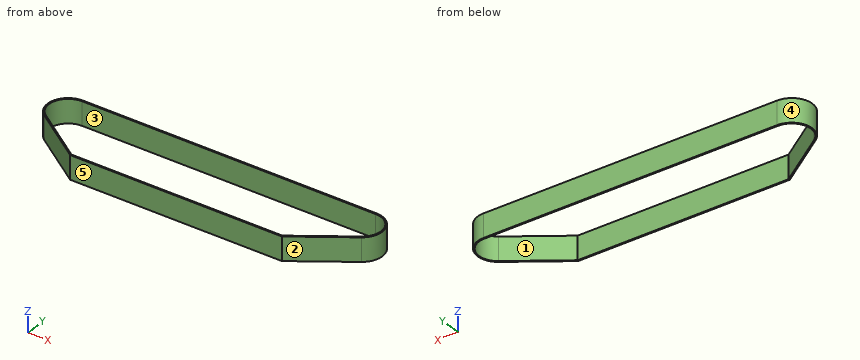
```python
from build123d import *

# Parameters (mm, degrees)
EXTRUDE_1_DEPTH = 35


with BuildPart() as part:
    # 草图1 → 拉伸-薄壁1 (new body)
    with BuildSketch(Plane.XY):
        with BuildLine():
            Line((237.450135309, -25.014851143), (158.628665481, -80))
            Line((158.628665481, -80), (-158.628665481, -80))
            Line((-158.628665481, -80), (-237.450135309, -25.014851143))
            ThreePointArc((-237.450135309, -25.014851143), (-249.09641696, 9.145956487), (-220, 30.5))
            Line((-220, 30.5), (220, 30.5))
            ThreePointArc((220, 30.5), (249.09641696, 9.145956487), (237.450135309, -25.014851143))
        make_face()
        with BuildLine():
            Line((236.305864141, -23.374533035), (158, -78))
            Line((158, -78), (-158, -78))
            Line((-158, -78), (-236.305864141, -23.374533035))
            ThreePointArc((-236.305864141, -23.374533035), (-247.188455192, 8.546221636), (-220, 28.5))
            Line((-220, 28.5), (220, 28.5))
            ThreePointArc((220, 28.5), (247.188455192, 8.546221636), (236.305864141, -23.374533035))
        make_face(mode=Mode.SUBTRACT)
    extrude(amount=EXTRUDE_1_DEPTH)


solid = part.part
```
Input: part model. Units: mm. Frame: model coordinates. Face numbers are marked on the shaded views. A direction names the side the tool comes from. Round coordinates to 2 decimals unless told otherwise and drop trailing zeros. Loops run counter-clockwise (first coordinate to the right, second up) from the corner with the lowest first, then second, coordinate; pieces in that order, holes last. Notation, with made-up numbers: (8, -6.75) -> (14, -6.75) arc R10 cw to (14, 12.25) -> close; hole circle Ø6 at (32.25, -7.75). An arc over 180 degrees is marked (long way). Write each question's results on one line, items separated by ' | '.
1. First-contact query: P1, Ø1, axis at y = -50, z = 18, coming from the -X side; P2, Ø1.5, axis at y = -44.5, z = 21, coming from the -X side; P3, Ø6, axis at y = -9, z = 25, coming from the -X side. Flat tips, straight axial feed; report the tip coordinate or a pass-through.
Geometry results:
P1: x = -202.35 | P2: x = -210.59 | P3: x = -249.9
2. Section A-A (x = 4). Return loops of the section in (y, z), and give its area (3 significant figures).
Geometry results:
outline: (-80, 0) -> (-78, 0) -> (-78, 35) -> (-80, 35) -> close; (28.5, 0) -> (30.5, 0) -> (30.5, 35) -> (28.5, 35) -> close | area: 140 mm2
3. Mould query, pull axis X, two halves, no side actions, for the marked faces 3, 4 and 5. Classes: +X half, -X half, draft (parallel to the pull), parting line (faces both ways), or undercut.
Geometry results:
face 3: undercut | face 4: -X half | face 5: draft
4. Section B-B (y = -57). Return loops of the section in (x, z), and give its area (3 significant figures).
Geometry results:
outline: (-191.6, 0) -> (-188.1, 0) -> (-188.1, 35) -> (-191.6, 35) -> close; (188.1, 0) -> (191.6, 0) -> (191.6, 35) -> (188.1, 35) -> close | area: 245 mm2
5. Set-up query: the marked faces 1 and 2. Return all of +Z, -Z, +X, -X, +Y, -Y with unobstructed straight access to the full face (end or side cutting, diameter ignored); none if empty.
Geometry results:
face 1: +Z, -Z | face 2: +Z, -Z, +X, -Y
6. Ray query, line 1 (Y direction, x = 29, z = 7); line 2 (X direction, y = 2, z = 15); line 3 (Y direction, x = 174.5, z = 33.5). Return the intervals inside material, ascending. Write a range as from..to.
Geometry results:
line 1: -80..-78, 28.5..30.5 | line 2: -250.43..-248.43, 248.43..250.43 | line 3: -68.93..-66.49, 28.5..30.5
7. Section C-C (z = 9.5). Return loops of the section in (x, y), and give its area (3 significant figures).
Geometry results:
outline: (-237.45, -25.01) -> (-158.63, -80) -> (158.63, -80) -> (237.45, -25.01) arc R30.5 ccw to (220, 30.5) -> (-220, 30.5) arc R30.5 ccw to start; hole (-236.31, -23.37) -> (-158, -78) -> (158, -78) -> (236.31, -23.37) arc R28.5 ccw to (220, 28.5) -> (-220, 28.5) arc R28.5 ccw to start | area: 2,200 mm2
